```python
from build123d import *

# Parameters (mm, degrees)
SKETCH1_W           = 35
SKETCH1_H           = 20
SKETCH1_R           = 2.5
BOSS_EXTRUDE1_DEPTH = 13
SKETCH2_R           = 4
CUT_EXTRUDE1_DEPTH  = 30.584624385


with BuildPart() as part:
    # Sketch1 → Boss-Extrude1 (new body)
    with BuildSketch(Plane(origin=(0, 0, 0), x_dir=(1, 0, 0), z_dir=(0, 1, 0))):
        Rectangle(SKETCH1_W, SKETCH1_H)
        with Locations(Location((-10, 0, 0), (0, 0, 270))):
            Circle(SKETCH1_R, mode=Mode.SUBTRACT)
        with Locations(Location((10, 0, 0), (0, 0, 270))):
            Circle(SKETCH1_R, mode=Mode.SUBTRACT)
    extrude(amount=BOSS_EXTRUDE1_DEPTH)

    # Sketch2 → Cut-Extrude1 (cut, through all)
    with BuildSketch(Plane.XY.offset(10)):
        with Locations((0, 6.5)):
            Circle(SKETCH2_R)
    extrude(amount=-CUT_EXTRUDE1_DEPTH, mode=Mode.SUBTRACT)


solid = part.part
```
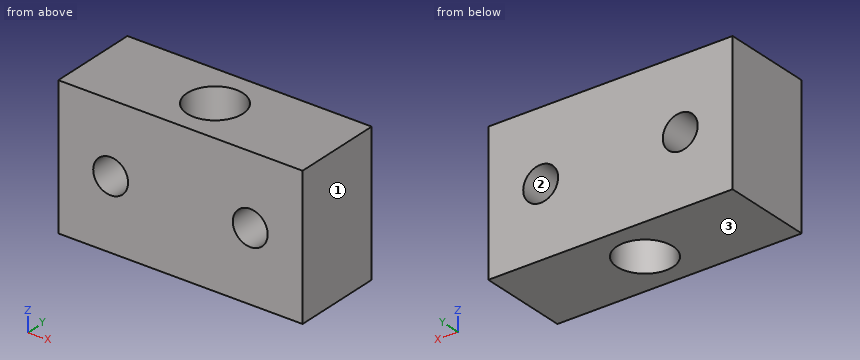
Can you work these out from the model? Positions are in its coordinate system, mm. Face numbers are marked on the shaded views. Give positions to 0.01 mm unless a question says otherwise; leave off trailing zeros. Write each loop counter-clockwise with the first axis right and the second up, starting at its lowest first coordinate (ties: lowest second). Pieces come first, ordered by that corner, then holes. Notation, with made-up numbers: (-34, 24) -> (-27, 24) arc R15 ccw to (-27, 50) -> close; hole circle Ø10 at (5.25, -3.75). An arc over 180 degrees is marked (long way). One line per item, written item: value.
Q1. Please list where these lines run through material, in increasing order: line 1 (Y direction, x = 0, z = -2.75); line 2 (X direction, y = 7, z = 0.75); line 3 (X direction, y = 9.5, z = 0). Write a range as [from, to].
Results found:
line 1: y = [0, 2.5], [10.5, 13]
line 2: x = [-17.5, -12.38], [-7.62, -3.97], [3.97, 7.62], [12.38, 17.5]
line 3: x = [-17.5, -12.5], [-7.5, -2.65], [2.65, 7.5], [12.5, 17.5]
Q2. Imagine slicing it at A-A on z = 0. Please give me the cut outline in (x, y).
Results found:
outline: (-17.5, 0) -> (-12.5, 0) -> (-12.5, 13) -> (-17.5, 13) -> close; (-7.5, 0) -> (7.5, 0) -> (7.5, 13) -> (-7.5, 13) -> close; (12.5, 0) -> (17.5, 0) -> (17.5, 13) -> (12.5, 13) -> close; hole circle Ø8 at (0, 6.5)
Q3. We'd pull the mould along X, two halves only. Please class the marked faces 1, 2 and 3: +X half, -X half, draft (parallel to the pull), parting line (faces both ways), or undercut.
Results found:
face 1: +X half
face 2: undercut
face 3: draft
Q4. Imagine slicing it at C-C on y = 6. Please give me the cut outline in (x, z).
Results found:
outline: (-17.5, -10) -> (-3.97, -10) -> (-3.97, 10) -> (-17.5, 10) -> close; (3.97, -10) -> (17.5, -10) -> (17.5, 10) -> (3.97, 10) -> close; hole circle Ø5 at (-10, 0); hole circle Ø5 at (10, 0)
Q5. Imagine slicing it at D-D on z = 8. Please give me the cut outline in (x, y).
Results found:
outline: (-17.5, 0) -> (17.5, 0) -> (17.5, 13) -> (-17.5, 13) -> close; hole circle Ø8 at (0, 6.5)
Q6. Imagine slicing it at B-B on x = 10. Please give me the cut outline in (y, z), and give its area (3 significant figures).
Results found:
outline: (0, -10) -> (13, -10) -> (13, -2.5) -> (0, -2.5) -> close; (0, 2.5) -> (13, 2.5) -> (13, 10) -> (0, 10) -> close
area: 195 mm^2
